from build123d import *

# Parameters (mm, degrees)
F1_DEPTH  = 25.4
F2_W      = 25.4
F2_H      = 3.175
F3_DEPTH  = 25.4
F4_W      = 25.4
F4_H      = 3.175
F5_DEPTH  = 25.4
F7_DEPTH  = 25.4
F8_DEPTH  = 6.35
F10_DEPTH = 6.35
F13_DEPTH = 19.05


with BuildPart() as f1:
    # F0 (on Front) → F1 (new body)
    with BuildSketch(Plane.XZ):
        with BuildLine():
            Line((246.660952732, 12.7), (-134.339047268, 12.7))
            Line((-134.339047268, 12.7), (-134.339047268, -12.7))
            Line((-134.339047268, -12.7), (-76.4309399312, -12.7))
            ThreePointArc((-76.4309399312, -12.7), (56.160952732, 0), (188.7528453951, -12.7))
            Line((188.7528453951, -12.7), (246.660952732, -12.7))
            Line((246.660952732, -12.7), (246.660952732, 12.7))
        make_face()
    extrude(amount=F1_DEPTH)

    # F2 (on face) → F3 (cut)
    with BuildSketch(Plane.YZ.offset(246.660952732)):
        with Locations((-12.7, 0)):
            Rectangle(F2_W, F2_H)
    extrude(amount=-F3_DEPTH, mode=Mode.SUBTRACT)

    # F4 (on face) → F5 (cut)
    with BuildSketch(Plane(origin=(-134.339047268, 0, 0), x_dir=(0, -1, 0), z_dir=(-1, 0, 0))):
        with Locations((12.7, 0)):
            Rectangle(F4_W, F4_H)
    extrude(amount=-F5_DEPTH, mode=Mode.SUBTRACT)

    # F6 (on face) → F7 (cut)
    with BuildSketch(Plane.XY.offset(12.7)):
        Polygon((-134.339047268, 0), (-134.339047268, -25.4), (-121.639047268, -12.7), (-108.939047268, 0), align=None)
        Polygon((233.960952732, -12.7), (246.660952732, -25.4), (246.660952732, 0), (221.260952732, 0), align=None)
    extrude(amount=-F7_DEPTH, mode=Mode.SUBTRACT)

    # F6 (on face) → F8 (cut)
    with BuildSketch(Plane.XY.offset(12.7)):
        Polygon((-108.939047268, 0), (-121.639047268, -12.7), (233.960952732, -12.7), (221.260952732, 0), align=None)
    extrude(amount=-F8_DEPTH, mode=Mode.SUBTRACT)

    # F9 (on face) → F10 (cut)
    with BuildSketch(Plane.XY.offset(6.35)):
        Polygon((-0.989047268, 0), (-13.689047268, 0), (-20.039047268, -12.7), (5.360952732, -12.7), align=None)
        Polygon((126.010952732, 0), (113.310952732, 0), (106.960952732, -12.7), (132.360952732, -12.7), align=None)
    extrude(amount=-F10_DEPTH, mode=Mode.SUBTRACT)

    # F11 (on face) + F12 (on face) → F13 (cut)
    with BuildSketch(Plane(origin=(0, 0, -12.7), x_dir=(1, 0, 0), z_dir=(0, 0, -1))):
        with BuildLine():
            ThreePointArc((-116.3785350259, 19.5480122421), (-117.8451937838, 18.568022191), (-117.501067041, 16.837980227))
            Line((-117.501067041, 16.837980227), (-116.3785350259, 17.9605122421))
            Line((-116.3785350259, 17.9605122421), (-116.3785350259, 19.5480122421))
        make_face()
        with BuildLine():
            Line((-116.3785350259, 17.9605122421), (-114.7910350259, 17.9605122421))
            ThreePointArc((-114.7910350259, 17.9605122421), (-115.2560030108, 19.0830442573), (-116.3785350259, 19.5480122421))
            Line((-116.3785350259, 19.5480122421), (-116.3785350259, 17.9605122421))
        make_face()
        with BuildLine():
            ThreePointArc((-117.501067041, 16.837980227), (-115.771025077, 16.4938534843), (-114.7910350259, 17.9605122421))
            Line((-114.7910350259, 17.9605122421), (-116.3785350259, 17.9605122421))
            Line((-116.3785350259, 17.9605122421), (-117.501067041, 16.837980227))
        make_face()
    with BuildSketch(Plane(origin=(0, 0, -12.7), x_dir=(1, 0, 0), z_dir=(0, 0, -1))):
        with BuildLine():
            Line((228.7004404898, 17.9605122421), (229.822972505, 16.837980227))
            ThreePointArc((229.822972505, 16.837980227), (230.1670992477, 17.3530022933), (230.2879404898, 17.9605122421))
            ThreePointArc((230.2879404898, 17.9605122421), (229.822972505, 19.0830442573), (228.7004404898, 19.5480122421))
            Line((228.7004404898, 19.5480122421), (228.7004404898, 17.9605122421))
        make_face()
        with BuildLine():
            ThreePointArc((228.7004404898, 19.5480122421), (227.5779084747, 19.0830442573), (227.1129404898, 17.9605122421))
            Line((227.1129404898, 17.9605122421), (228.7004404898, 17.9605122421))
            Line((228.7004404898, 17.9605122421), (228.7004404898, 19.5480122421))
        make_face()
        with BuildLine():
            Line((228.7004404898, 17.9605122421), (227.1129404898, 17.9605122421))
            ThreePointArc((227.1129404898, 17.9605122421), (228.0929305409, 16.4938534843), (229.822972505, 16.837980227))
            Line((229.822972505, 16.837980227), (228.7004404898, 17.9605122421))
        make_face()
    extrude(amount=-F13_DEPTH, mode=Mode.SUBTRACT)


solid = f1.part
Input: part model. Units: mm. Frame: model coordinates. A direction names the side the tool comes from. Give positions to 0.01 mm unless a question says otherwise; leave off trailing zeros. Loops run counter-clockwise (first coordinate to the right, second up) from the corner with the lowest first, then second, coordinate; pieces in that order, holes last. Notation, with made-up numbers: M 3.5,-40 L 10.5,-40 A12 cw 10.5,-20 Z; hole C -30,9 d1. An arc over 180 degrees is marked long. Use one line per item in the form item = value.
1. Line query: L1, parallel to Z at x = -110.5, y = -7.25; L2, parallel to Z at x = 61.5, y = -22; L3, parallel to Z at x = -80, y = -12.25. Output: solid intervals per line, ascending.
Numbers:
L1 = -12.7 to -1.59, 1.59 to 6.35
L2 = -0.02 to 12.7
L3 = -12.7 to 6.35
2. Section query A-A, the plane z = -7.5. Return the cut outline in (x, y) (1 decimal), and give its area (3 significant figures).
Numbers:
outline = M -134.3,-25.4 L -45.9,-25.4 L -45.9,0 L -108.9,0 Z; M 158.2,-25.4 L 246.7,-25.4 L 221.3,0 L 158.2,0 Z; hole C -116.4,-18 d3.2; hole C 228.7,-18 d3.2
area = 3,830 mm²
3. Section query C-C, the plane y = -8.5. Return the cut outline in (x, z).
Numbers:
outline = M -117.44,-12.7 L -76.43,-12.7 A698.5 cw 188.75,-12.7 L 229.76,-12.7 L 229.76,-1.59 L 221.26,-1.59 L 221.26,1.59 L 229.76,1.59 L 229.76,6.35 L 130.26,6.35 L 130.26,0 L 109.06,0 L 109.06,6.35 L 3.26,6.35 L 3.26,0 L -17.94,0 L -17.94,6.35 L -117.44,6.35 L -117.44,1.59 L -108.94,1.59 L -108.94,-1.59 L -117.44,-1.59 Z
4. Section query D-D, the plane x = -8.5. Return the cut outline in (y, z).
Numbers:
outline = M -25.4,-3 L 0,-3 L 0,0 L -12.7,0 L -12.7,12.7 L -25.4,12.7 Z
5. Reachability of faces 4 (the face through (55, -6, 6.35)), 5 (the face through (-116, -15, 1.588)), 6 (the face through (-8, -8, 0)) from +Z, -Z, +X, -X, +Y, -Y: full face, straight path, thin tool, end or side. Return the list, or none.
Numbers:
face_4 = +Z, +X, -X, +Y
face_5 = -X, +Y, -Y
face_6 = +Z
6. Pull-direction query (X, two-part tool) for faces 1 (the face through (129.23, -6.44, 3.22)), 2 (the face through (228, -16, -1.588)), 3 (the face through (-121.82, -12.88, -7.07)); classes: released by +X, released by -X, zero draft, split by the parting line, or undercut.
Numbers:
face_1 = undercut
face_2 = zero draft
face_3 = released by -X
7. First-contact query: pin 1 (3 mm diameter, centred on y = -6.5, z = -3.5, fed in from +X); pin 2 (6.5 mm diameter, centred on x = 50.5, y = -4, fed in from +Z); pin 3 (6.5 mm diameter, centred on x = 116, y = -7.5, fed in from +Z). Flat tips, straight axial feed; report the tip coordinate or a pass-through.
Numbers:
pin_1 = 229.26
pin_2 = 6.35
pin_3 = 0
8. Section query B-B, the plane x = 218. Return the cut outline in (y, z), and give its area (3 significant figures).
Numbers:
outline = M -25.4,-12.7 L 0,-12.7 L 0,6.35 L -12.7,6.35 L -12.7,12.7 L -25.4,12.7 Z
area = 565 mm²
